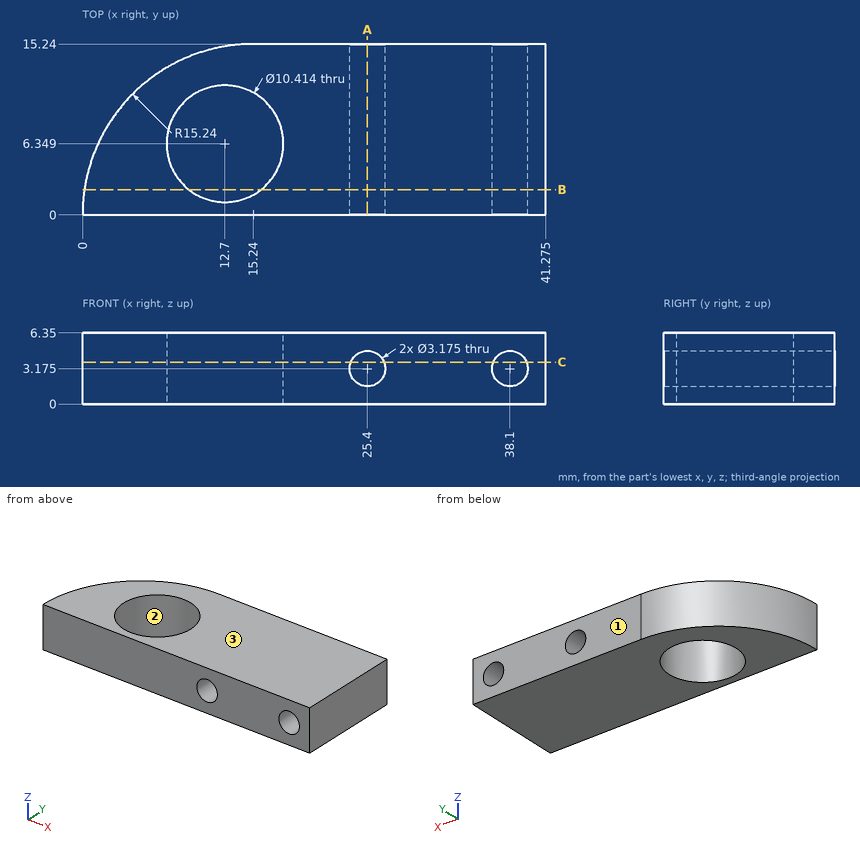
The figure shows three views and two pictorial views of one solid part (mm, origin at its lowest corner). Answer the questions. Give positions to 0.01 mm unless a question says otherwise; leave off trailing zeros. Loops run counter-clockwise (first coordinate to the right, second up) from the corner with the lowest first, then second, coordinate; pieces in that order, holes last. Notation, with made-up numbers: (39, -12.5) -> (93, -12.5) arc R30 ccw to (93, 16.5) -> close; hole circle Ø10 at (-33, 78). An arc over 180 degrees is marked (long way). Use a Markdown table: item, result. Add a question column.
1. Determine the mould class of the marked faces 1, 2 and 3 for opening direction Y: released by +Y, released by -Y, zero draft, split by the parting line, or undercut.
2. Section B-B on y = 2.25 is taken. State how many separate pieces and enclosed holes the cut face has, and give its area (3 significant figures).
3. A flat-ended cylindrical pin translates along its axis: pin 1 Ø3.5 at (x, z) = (38.1, 3.175) entering from -Y. Find the tip coordinate at first contact, or state that the pin passes through.
4. Find the intervals of material crossed by probe 1 along X at (y, z) = (7.75, 4) (3 decimals); probe 2 along Z at (x, y) = (38.1, 7.25); probe 3 along X at (y, z) = (10.25, 4) (1 decimal), in increasing order.
5. Section A-A on x = 25.4 is taken. Determine the outline of the cut face in (y, z), and give its area (3 significant figures).
6. Section C-C on z = 3.75 is taken. Determine the outline of the cut face in (x, y) (3 decimals).
Results below:
| question | item | result |
|---|---|---|
| 1 | face 1 | released by +Y |
| 1 | face 2 | undercut |
| 1 | face 3 | zero draft |
| 2 | separate pieces | 2 |
| 2 | enclosed holes | 2 |
| 2 | area | 204 mm^2 |
| 3 | pin 1 | stops at y = 0 |
| 4 | probe 1 | x = 2.118 to 7.685, 17.715 to 24.044, 26.756 to 36.744, 39.456 to 41.275 |
| 4 | probe 2 | z = 0 to 1.59, 4.76 to 6.35 |
| 4 | probe 3 | x = 4 to 9.3, 16.1 to 24, 26.8 to 36.7, 39.5 to 41.3 |
| 5 | outline | (0, 0) -> (15.24, 0) -> (15.24, 1.59) -> (0, 1.59) -> close; (0, 4.76) -> (15.24, 4.76) -> (15.24, 6.35) -> (0, 6.35) -> close |
| 5 | area | 48.4 mm^2 |
| 6 | outline | (0, 0) -> (23.92, 0) -> (23.92, 15.24) -> (15.24, 15.24) arc R15.24 ccw to start; (26.88, 0) -> (36.62, 0) -> (36.62, 15.24) -> (26.88, 15.24) -> close; (39.58, 0) -> (41.275, 0) -> (41.275, 15.24) -> (39.58, 15.24) -> close; hole circle Ø10.414 at (12.7, 6.349) |
